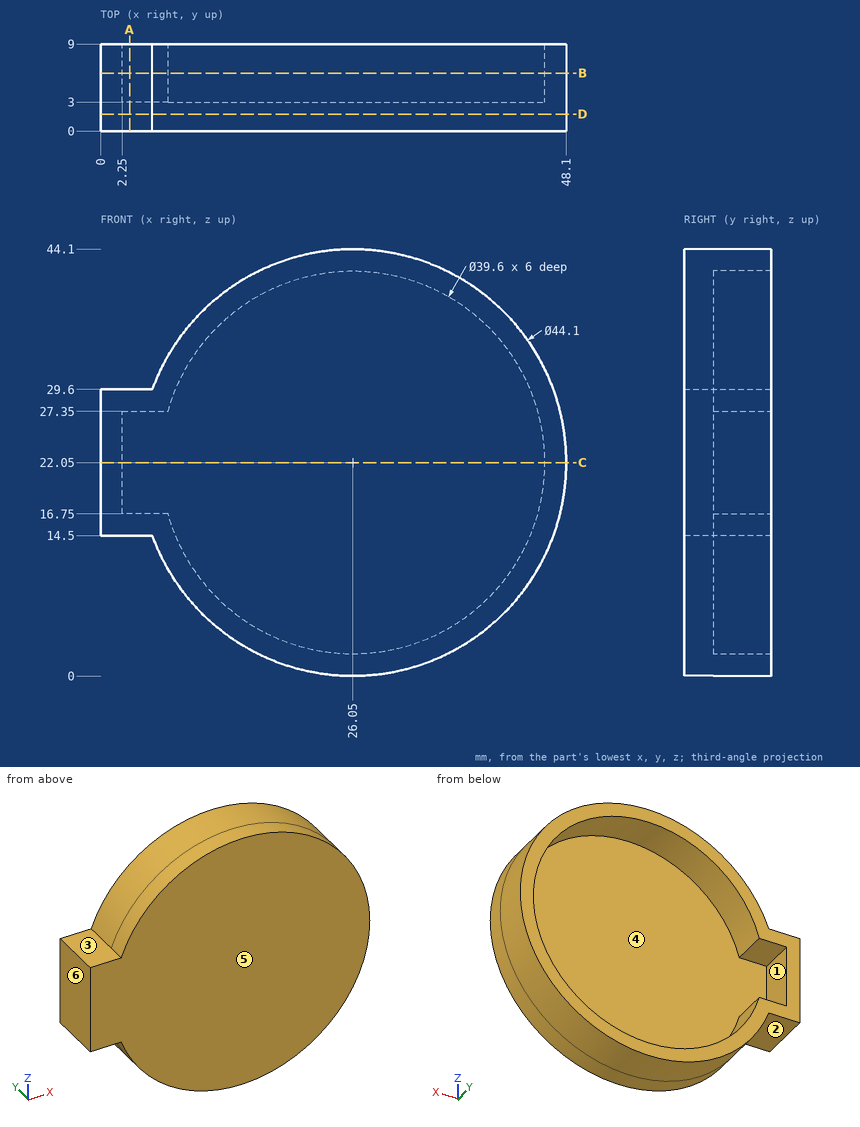
Study the drawing (mm; zero at the part's minimum x, y, z) and answer. A direction names the side the tool comes from. Give positions to 0.01 mm unless a question says otherwise; leave off trailing zeros. Write each loop counter-clockwise with the first axis right and the second up, starting at its lowest first coordinate (ties: lowest second). Pieces come first, ordered by that corner, then holes. Notation, with made-up numbers: (45.25, 84.5) - (62.25, 84.5) arc R14 cw to (62.25, 104.5) - close; hole circle Ø7 at (-15.75, 84.25). An arc over 180 degrees is marked (long way). Use a Markdown table: item, result.
1. Section C-C on z = 22.05 is taken. Write down the section's boundary in (x, y), plus the area to 3 significant figures.
Values follow:
| item | result |
|---|---|
| outline | (0, 0) - (48.1, 0) - (48.1, 9) - (45.85, 9) - (45.85, 3) - (2.25, 3) - (2.25, 9) - (0, 9) - close |
| area | 171 mm² |
2. A tool of negligible diameter and unlimited length cuts with its end or side. For the marked faces 1, 2 and 3, from which of +Z, -Z, +X, -X, +Y, -Y can it reach the whole face along a straight path? Write none if from no direction.
Values follow:
| item | result |
|---|---|
| face 1 | +Y |
| face 2 | -Z, -X, +Y, -Y |
| face 3 | +Z, -X, +Y, -Y |
3. Section D-D on y = 1.75 is taken. Write down the section's boundary in (x, z).
Values follow:
| item | result |
|---|---|
| outline | (0, 14.5) - (5.33, 14.5) arc R22.05 ccw (long way) to (5.33, 29.6) - (0, 29.6) - close |
4. Section B-B on y = 6 is taken. Write down the section's boundary in (x, z).
Values follow:
| item | result |
|---|---|
| outline | (0, 14.5) - (5.33, 14.5) arc R22.05 ccw (long way) to (5.33, 29.6) - (0, 29.6) - close; hole (2.25, 16.75) - (6.97, 16.75) arc R19.8 ccw (long way) to (6.97, 27.35) - (2.25, 27.35) - close |
5. Find the intervals of material crossed by probe 1 along X at (y, z) = (6.35, 22.05); probe 2 along Z at (x, y) = (26.05, 6.85); probe 3 along Y at (x, z) = (35.5, 18), in increasing order. Write a range as from..to.
Values follow:
| item | result |
|---|---|
| probe 1 | x = 0..2.25, 45.85..48.1 |
| probe 2 | z = 0..2.25, 41.85..44.1 |
| probe 3 | y = 0..3 |
6. Each of these flat-tipped pins is pushed along its axis until it touches: P1, Ø4.5, axis at x = 2.5, y = 5, coming from the -Z side; P2, Ø4, axis at y = 8, z = 37.5, coming from the +X side; P3, Ø1, axis at x = 8.5, y = 5.5, coming from the -Z side. Where does it stop, or does it pass through?
Values follow:
| item | result |
|---|---|
| P1 | stops at z = 14.5 |
| P2 | stops at x = 43.52 |
| P3 | stops at z = 8.07 |
7. Section A-A on x = 3 is taken. Write down the section's boundary in (y, z), plus the area to 3 significant figures.
Values follow:
| item | result |
|---|---|
| outline | (0, 14.5) - (9, 14.5) - (9, 16.75) - (3, 16.75) - (3, 27.35) - (9, 27.35) - (9, 29.6) - (0, 29.6) - close |
| area | 72.3 mm² |
8. For a pull along X with two mould halves and no side action, classify the marked faces 4, 5 and 6 as released by +X, released by -X, zero draft, split by the parting line, or undercut.
Values follow:
| item | result |
|---|---|
| face 4 | undercut |
| face 5 | zero draft |
| face 6 | released by -X |
